Could you check a few things on this model? Use its own coordinates, in mm. A direction names the side the tool comes from. Round coordinates to 2 decimals unless told otherwise and drop trailing zeros. Write each loop counter-clockwise with the first axis right and the second up, starting at its lowest first coordinate (ties: lowest second). Pieces come first, ordered by that corner, then holes. Notation, with made-up numbers: M 62.25,73 L 94.25,73 A25 cw 94.25,92 Z; hole C 15.5,-30 d8. An arc over 180 degrees is marked long. One line per item, written item: value. Start each with the question number.
(1) Which directions (+Z, -Z, +X, -X, +Y, -Y) give clear straight access to the entire face, cutting with the end or side of a thin tool? Please do faces 1 (the face through (-6.503, -0.106, 0.806)), 2 (the face through (-7.366, 0, 0)), 3 (the face through (6.527, -0.106, 0.806)).
(2) I want a section at A-A on x = -0.25. Please give me the cut outline in (y, z), and give its area (3 significant figures).
(3) If I drill on L1, parallel to X at y = 1, z = 3.75; L2, parallel to Y at x = -1.75, z = 3.5; L3, parallel to Y at x = 3.25, z = 2.5, over which ranges is the centre line in solid material (lowest first)?
(4) I want a section at B-B on x = 2.75. Please give me the cut outline in (y, z).
(5) Thinking about a two-plate mould opening in Z: for faces 4 (the face through (7.366, 0, 0)), 5 (the face through (-2.792, -0.994, -4.476)), which applies, released by +Z, released by -Z, zero draft, split by the parting line, or undercut?
(6) I'm going to push flat-ended pins straight in: pin 1 Ø3 at (x, z) = (3.5, 0.5) entering from -Y; pin 2 Ø4 at (y, z) = (-2.5, -1.5) entering from +X; pin 3 Ø5 at (x, y) = (2.5, -3) entering from +Z. Where does each tip first touch, or does it pass through?
Autodesk Inventor part; units mm, degrees
ref_plane "YZ Plane" through (0, 0, 0) normal (1, 0, 0) x (0, 1, 0)
ref_plane "XZ Plane" through (0, 0, 0) normal (0, 1, 0) x (-1, 0, 0)
ref_plane "XY Plane" through (0, 0, 0) normal (0, 0, 1) x (1, 0, 0)
sketch "Sketch1" plane through (0, 0, 0) normal (0, 0, 1) x (1, 0, 0)
  line L0 (-7.366, 0) -> (7.366, 0)
  line L1 (-7.366, 0) -> (-7.366, 0.8128)
  line L2 (-7.366, 0.8128) -> (-5.6642, 0.8128)
  line L3 (-5.6642, 0.8128) -> (-5.6642, 4.5466)
  line L4 (-5.6642, 4.5466) -> (0, 4.6228)
  line L5 (0, 4.6228) -> (5.6642, 4.5466)
  line L6 (5.6642, 4.5466) -> (5.6642, 0.8128)
  line L7 (5.6642, 0.8128) -> (7.366, 0.8128)
  line L8 (7.366, 0.8128) -> (7.366, 0)
  point P0 (0, 0)
  point P1 (0, 0)
  dimension "d0" = 14.732
  dimension "d1" = 0.8128
  dimension "d2" = 4.6228
  dimension "d3" = 4.5466
  dimension "d4" = 11.3284
  dimension "d5" = 1.7018
  dimension "d6" = 1.7018
revolve "Revolution1" add sketch "Sketch1" angle 360 about axis through (-7.366, 0, 0) along (1, 0, 0)
equation "\"d5\" = d6"
properties part number "Flexiwheel Roller" material "PPS Plastic"
Found:
1. face 1: -X
1. face 2: +Z, -Z, -X, +Y, -Y
1. face 3: +X
2. outline: C 0,0 d9.24
2. area: 67.0 mm²
3. L1: x = -5.66 to 5.66
3. L2: y = -2.98 to 2.98
3. L3: y = -3.84 to 3.84
4. outline: C 0,0 d9.17
5. face 4: zero draft
5. face 5: split by the parting line
6. pin 1: stops at y = -4.59
6. pin 2: stops at x = 5.66
6. pin 3: stops at z = 4.56
